Autodesk Inventor part; units mm, degrees
ref_plane "YZ Plane" through (0, 0, 0) normal (1, 0, 0) x (0, 1, 0)
ref_plane "XZ Plane" through (0, 0, 0) normal (0, 1, 0) x (-1, 0, 0)
ref_plane "XY Plane" through (0, 0, 0) normal (0, 0, 1) x (1, 0, 0)
sketch "Sketch1" plane through (0, 0, 0) normal (0, 0, 1) x (1, 0, 0)
  line L0 (-6.9396, 11.6683) -> (6.9396, 11.6683)
  line L1 (6.9396, 11.6683) -> (6.9396, 0)
  line L2 (6.9396, 0) -> (-6.9396, 0)
  line L3 (-6.9396, 0) -> (-6.9396, 11.6683)
  circle A0 centre (0, 11.6683) radius 3.8335
  circle A1 centre (0, 11.6683) radius 2.9035
  point P0 (0, 0)
  point P1 (0, 0)
  point P2 (3.8335, 11.6683)
  point P3 (-3.8335, 11.6683)
extrude "Extrusion1" add sketch "Sketch1" along normal blind 2 contours A1 L0 A0 | L0 A0 A1 | L0 L1 L2 L3 A0
sketch "Sketch2" plane through (0, 0, 0) normal (0, 0, 1) x (1, 0, 0)
  line L0 (-6.9396, 11.6683) -> (-6.9396, 0)
  line L1 (-6.9396, 0) -> (6.9396, 0)
  line L2 (6.9396, 0) -> (6.9396, 4.5855)
  line L3 (6.9396, 4.5855) -> (-6.9396, 4.5855)
  line L4 (-6.9396, 4.5855) -> (-6.9396, 0)
  line L5 (6.9396, 0) -> (6.9396, 11.6683)
  point P0 (0, 0)
extrude "Extrusion2" add sketch "Sketch2" along normal blind 10
properties part number "exercise2"
Model file for the job. Use its own axes, mm. A direction names the side the tool comes from. Round coordinates to 2 decimals unless told otherwise and drop trailing zeros. Loops run counter-clockwise (first coordinate to the right, second up) from the corner with the lowest first, then second, coordinate; pieces in that order, holes last.
1. Wall check: probe 1 along Y at (x, z) = (0, 0.9); probe 2 along Z at (x, y) = (5.75, 4.75); probe 3 along Y at (x, z) = (0.75, 8). Give the ranges that are in metal, low to high.
Check values:
probe 1: y = 0 to 8.76, 14.57 to 15.5
probe 2: z = 0 to 2
probe 3: y = 0 to 4.59
2. Band-saw the part on C-C, the plane x = -4.5. List the corners of the cut face in (y, z).
Check values:
outline: (0, 0) - (11.67, 0) - (11.67, 2) - (4.59, 2) - (4.59, 10) - (0, 10) - close
3. Band-saw the part on A-A, the plane x = 0. List the corners of the cut face in (y, z), and give its area (3 significant figures).
Check values:
outline: (0, 0) - (8.76, 0) - (8.76, 2) - (4.59, 2) - (4.59, 10) - (0, 10) - close; (14.57, 0) - (15.5, 0) - (15.5, 2) - (14.57, 2) - close
area: 56.1 mm2
4. Band-saw the part on B-B, the plane y = 12.5. List the corners of the cut face in (x, z).
Check values:
outline: (-3.74, 0) - (-2.78, 0) - (-2.78, 2) - (-3.74, 2) - close; (2.78, 0) - (3.74, 0) - (3.74, 2) - (2.78, 2) - close
5. Drop flat-ended pins along their axis: P1, Ø2, axis at x = 5.5, z = 1, coming from the +Y side; P2, Ø3.5, axis at x = 0, y = 11.67, coming from the +Z side; P3, Ø5.5, axis at x = 0, y = 10.5, coming from the +Z side. Give the stop position or say it passes through.
Check values:
P1: stops at y = 11.67
P2: passes through
P3: stops at z = 2
6. Band-saw the part on D-D, the plane z = 4.5. List the corners of the cut face in (x, y), and give its area (3 significant figures).
Check values:
outline: (-6.94, 0) - (6.94, 0) - (6.94, 4.59) - (-6.94, 4.59) - close
area: 63.6 mm2
7. Tool access for faces 4 (the flat face through (-5, 11.668, 1)), 5 (the flat face through (0, 4.586, 6)), 6 (the flat face through (5, 11.668, 1)), 7 (the flat face through (6.94, 3, 4)): list every direction of +Z, -Z, +X, -X, +Y, -Y with a clear straight run to the whole face (end or side of a thin tool).
Check values:
face 4: +Z, -Z, -X, +Y
face 5: +Z, +X, -X, +Y
face 6: +Z, -Z, +X, +Y
face 7: +Z, -Z, +X, +Y, -Y
8. Mould opens along Y. For faces 1 (the cylindrical face through (-0.38, 8.79, 0.99)), 2 (the flat face through (0, 0, 5)), 3 (the flat face through (0, 8, 2)) say: +Y half, -Y half, draft (parallel to the pull), parting line (faces both ways), or undercut.
Check values:
face 1: undercut
face 2: -Y half
face 3: draft
